Geometry: final body of the model. Coordinates: model frame, mm. A direction names the side the tool comes from. Give positions to 0.01 mm unless a question says otherwise; leave off trailing zeros. Loops run counter-clockwise (first coordinate to the right, second up) from the corner with the lowest first, then second, coordinate; pieces in that order, holes last. Notation, with made-up numbers: (84, 68) - (98, 68) arc R14 cw to (98, 91) - close; hole circle Ø9 at (49.5, 54). An arc over 180 degrees is marked (long way). Use one line per item in the form item = value.
Autodesk Inventor part; units mm, degrees
ref_plane "YZ Plane" through (0, 0, 0) normal (1, 0, 0) x (0, 1, 0)
ref_plane "XZ Plane" through (0, 0, 0) normal (0, 1, 0) x (-1, 0, 0)
ref_plane "XY Plane" through (0, 0, 0) normal (0, 0, 1) x (1, 0, 0)
sketch "Sketch1" plane through (0, 0, 0) normal (0, 1, 0) x (-1, 0, 0)
  line L0 (24.13, 54.61) -> (-24.13, 54.61)
  line L1 (-24.13, 54.61) -> (-24.13, -54.61)
  line L2 (-24.13, -54.61) -> (24.13, -54.61)
  line L3 (24.13, -54.61) -> (24.13, 54.61)
  point P0 (0, 0)
  dimension "d0" = 109.22
  dimension "d1" = 48.26
  dimension "d4" = 24.13
  dimension "d5" = 54.61
extrude "Extrusion1" add sketch "Sketch1" along normal blind 1.6
sketch "Sketch2" plane through (0, 1.6, 0) normal (0, 1, 0) x (1, 0, 0)
  line L0 (-13.716, 50.165) -> (-27.94, 50.165)
  line L1 (-27.94, 50.165) -> (-27.94, 35.179)
  line L2 (-27.94, 35.179) -> (-13.716, 35.179)
  line L3 (-13.716, 35.179) -> (-13.716, 50.165)
  line L4 (-24.13, 54.61) -> (-24.13, -54.61)
  line L5 (24.13, 54.61) -> (-24.13, 54.61)
  point P0 (0, 0)
  dimension "d6" = 14.224
  dimension "d7" = 14.986
  dimension "d8" = 3.81
  dimension "d9" = 4.445
extrude "Extrusion2" add sketch "Sketch2" along normal blind 6.35
sketch "Sketch3" plane through (0, 1.6, 0) normal (0, 1, 0) x (1, 0, 0)
  line L0 (-31.369, 1.778) -> (-13.589, 1.778)
  line L1 (-13.589, 1.778) -> (-13.589, 34.29)
  line L2 (-13.589, 34.29) -> (-31.369, 34.29)
  line L3 (-31.369, 34.29) -> (-31.369, 1.778)
  line L4 (24.13, 54.61) -> (-24.13, 54.61)
  line L5 (-24.13, 35.179) -> (-24.13, -54.61)
  point P0 (0, 0)
  dimension "d12" = 32.512
  dimension "d13" = 17.78
  dimension "d14" = 20.32
  dimension "d15" = 7.239
extrude "Extrusion3" add sketch "Sketch3" along normal blind 6.35
sketch "Sketch4" plane through (-31.369, 1.6, -34.29) normal (-1, 0, 0) x (0, 0, 1)
  line L0 (11.6254, 3.2104) -> (20.2625, 3.2104)
  line L1 (20.2625, 3.2104) -> (23.564, 8.9287)
  line L2 (23.564, 8.9287) -> (8.324, 8.9287)
  line L3 (8.324, 8.9287) -> (11.6254, 3.2104)
  point P0 (34.29, -1.6)
  dimension "d18" = 120
  dimension "d19" = 120
  dimension "d20" = 15.24
extrude "Extrusion4" add sketch "Sketch4" along normal blind 8.636 and the other way blind 4.318
fillet "Fillet1" radius 1.5875 4 edges at (-33.528, 10.5287, -25.966) (-33.528, 10.5287, -10.726) (-35.687, 4.8104, -22.6646) (-35.687, 4.8104, -14.0275)
properties part number "ControlBoard"
(1) Cut plane C-C (x = -20). Return the cut outline in (y, z) (3 decimals), plus the area to 3 significant figures.
Solution:
outline = (0, -54.61) - (1.6, -54.61) - (1.6, -50.165) - (7.95, -50.165) - (7.95, -35.179) - (1.6, -35.179) - (1.6, -34.29) - (7.95, -34.29) - (7.95, -1.778) - (1.6, -1.778) - (1.6, 54.61) - (0, 54.61) - close
area = 476 mm2
(2) Access query for faces 1 (the face through (-36, 4.81, -18)), 2 (the face through (-21, 5, -50.165)), 3 (the face through (-31.369, 4, -18)), 4 (the face through (-21, 5, -35.179)). Directions: +Z, -Z, +X, -X, +Y, -Y. A direction counts if a zero-diameter tool reaches every point of the face in a straight line with its end or side. Return the directions, or none.
Solution:
face_1 = +Z, -Z, -X, -Y
face_2 = -Z, +X, -X, +Y
face_3 = -X, -Y
face_4 = +X, -X, +Y
(3) Cut plane B-B (z = -18). Return the cut outline in (x, y) (3 decimals).
Solution:
outline = (-40.005, 4.81) - (-31.369, 4.81) - (-31.369, 1.6) - (-24.13, 1.6) - (-24.13, 0) - (24.13, 0) - (24.13, 1.6) - (-13.589, 1.6) - (-13.589, 7.95) - (-27.051, 7.95) - (-27.051, 10.529) - (-40.005, 10.529) - close
(4) Pin query (flat end, axial travel): P1, Ø3, axis at x = -25.5, y = 5.5, coming from the +Z side; P2, Ø12, axis at x = -13, z = 43, coming from the +Y side; P3, Ø8, axis at x = -28, z = -30, coming from the +Y side; P4, Ø5, axis at x = -5, z = -31, coming from the -Y side. Return the tip coordinate at first contact, or that it passes through.
Solution:
P1 = -1.78
P2 = 1.6
P3 = 7.95
P4 = 0
(5) Cut plane D-D (z = -43.5). Return the cut outline in (x, y), plus the area to 3 significant figures.
Solution:
outline = (-27.94, 1.6) - (-24.13, 1.6) - (-24.13, 0) - (24.13, 0) - (24.13, 1.6) - (-13.72, 1.6) - (-13.72, 7.95) - (-27.94, 7.95) - close
area = 168 mm2
(6) Cut plane A-A (y = 3.25). Return the cut outline in (x, z) (3 decimals), plus the area to 3 significant figures.
Solution:
outline = (-31.369, -34.29) - (-13.589, -34.29) - (-13.589, -1.778) - (-31.369, -1.778) - close; (-27.94, -50.165) - (-13.716, -50.165) - (-13.716, -35.179) - (-27.94, -35.179) - close
area = 791 mm2
(7) Material intervals for L1, parallel to Z at x = -25, y = 7.5 (3 decimals); L2, parallel to Y at x = -23.5, z = -21; L3, parallel to Y at x = 17, z = 7.5, sorted ascending. Write a range as from..to.
Solution:
L1 = -50.165..-35.179, -34.29..-1.778
L2 = 0..7.95
L3 = 0..1.6
